Read the model definition and answer for the solid it produces. Units are mm, in the model's axes. Coordinates: 2 decimals unless noted, no trailing zeros. Write each loop counter-clockwise with the first axis right and the second up, starting at its lowest first coordinate (ties: lowest second). Pieces come first, ordered by that corner, then holes. Notation, with made-up numbers: (76, -10.75) -> (89, -10.75) arc R17 ccw to (89, 16.25) -> close; hole circle Ø8 at (83.5, 24.25). An arc over 180 degrees is marked (long way). One line per item, written item: value. Start each with the question number.
1. Find section C-C, the plane z = 15.5. Write down the section's boundary in (x, y).
2. Find section D-D, the plane y = 42.96. Write down the section's boundary in (x, z).
3. Find section B-B, the plane y = 51. Write down the section's boundary in (x, z).
4. Find section A-A, the plane x = 80. Write down the section's boundary in (y, z), and give its area (3 significant figures).
5. Consider line 1 along Y through (x, z) = (20, 9.75); line 2 along X through (y, z) = (51.5, 7.5); line 3 along X through (y, z) = (54, 4). Determine where each line is inside the solid, lowest interval first.
6. For a pull along Y with two mould halves and no side action, classify faces 1 (the flat face through (23, 61, 9)), 2 (the flat face through (49, 31, 0)), 3 (the cylindrical face through (29.412, 60.527, 9.126)) as pulls with the +Y half, pulls with the -Y half, needs draft (parallel to the pull), parting line crosses it, or undercut.
Autodesk Inventor part; units mm, degrees
ref_plane "YZ Plane" through (0, 0, 0) normal (1, 0, 0) x (0, 1, 0)
ref_plane "XZ Plane" through (0, 0, 0) normal (0, 1, 0) x (-1, 0, 0)
ref_plane "XY Plane" through (0, 0, 0) normal (0, 0, 1) x (1, 0, 0)
sketch "Boceto1" plane through (0, 0, 0) normal (0, 0, 1) x (1, 0, 0)
  line L0 (0, 0) -> (100, 0)
  line L1 (100, 0) -> (100, 61)
  line L2 (100, 61) -> (0, 61)
  line L3 (0, 61) -> (0, 0)
  dimension "d0" = 61
  dimension "d1" = 100
extrude "Extrusión1" add sketch "Boceto1" along normal blind 18
sketch "Boceto2" plane through (0, 0, 18) normal (0, 0, 1) x (1, 0, 0)
  circle A0 centre (50, 51) radius 11
  line L0 (0, 61) -> (0, 0)
  line L1 (100, 61) -> (0, 61)
  line L2 (50, 51) -> (20, 51) construction
  circle A1 centre (20, 51) radius 4
  line L3 (50, 51) -> (50, 22.8333) construction
  circle A2 centre (80, 51) radius 4
  circle A3 centre (29.6074, 59.04) radius 1.5
  line L4 (29.6074, 59.04) -> (50, 51) construction
  line L5 (50, 51) -> (78.7272, 39.674) construction
  circle A4 centre (70.3926, 42.96) radius 1.5
  line L6 (50, 51) -> (39.3624, 24.0188) construction
  circle A5 centre (41.96, 30.6074) radius 1.5
  line L7 (50, 51) -> (25.0918, 40.1786)
  line L8 (50, 51) -> (59.4119, 29.3362)
  point P0 (54.5826, 61)
  point P1 (45.4174, 61)
  dimension "d4" = 22
  dimension "d5" = 50
  dimension "d6" = 10
  dimension "d7" = 8
  dimension "d8" = 30
  dimension "d9" = 3
  dimension "d10" = 1.96
  dimension "d12" = 3
  dimension "d13" = 90
  dimension "d14" = 3
  dimension "d17" = 45
  dimension "d18" = 15.5
  dimension "d19" = 15.5
  dimension "d20" = 45
  dimension "d21" = 15.5
extrude "Extrusión2" cut sketch "Boceto2" against normal blind 18 contours A0 L8 L7 L1 | A0 L7 L8 | A1 | A2 | A3 | A4 | A5
properties part number "012" material "CFRP"
Answer block:
1. outline: (0, 0) -> (100, 0) -> (100, 61) -> (54.58, 61) arc R11 cw (long way) to (45.42, 61) -> (0, 61) -> close; hole circle Ø8 at (20, 51); hole circle Ø3 at (29.61, 59.04); hole circle Ø3 at (41.96, 30.61); hole circle Ø3 at (70.39, 42.96); hole circle Ø8 at (80, 51)
2. outline: (0, 0) -> (42.49, 0) -> (42.49, 18) -> (0, 18) -> close; (57.51, 0) -> (68.89, 0) -> (68.89, 18) -> (57.51, 18) -> close; (71.89, 0) -> (100, 0) -> (100, 18) -> (71.89, 18) -> close
3. outline: (0, 0) -> (16, 0) -> (16, 18) -> (0, 18) -> close; (24, 0) -> (39, 0) -> (39, 18) -> (24, 18) -> close; (61, 0) -> (76, 0) -> (76, 18) -> (61, 18) -> close; (84, 0) -> (100, 0) -> (100, 18) -> (84, 18) -> close
4. outline: (0, 0) -> (47, 0) -> (47, 18) -> (0, 18) -> close; (55, 0) -> (61, 0) -> (61, 18) -> (55, 18) -> close
4. area: 954 mm2
5. line 1: y = 0 to 47, 55 to 61
5. line 2: x = 0 to 16.03, 23.97 to 39.01, 60.99 to 76.03, 83.97 to 100
5. line 3: x = 0 to 17.35, 22.65 to 39.42, 60.58 to 77.35, 82.65 to 100
6. face 1: pulls with the +Y half
6. face 2: needs draft
6. face 3: undercut
